```python
from build123d import *

# Parameters (mm, degrees)
F1_DEPTH = 13
F2_R     = 3


with BuildPart() as f1:
    # F0 (on Top) → F1 (new body)
    with BuildSketch(Plane.XY):
        with BuildLine():
            ThreePointArc((11.590273, 26.810686), (0, 6.40625), (-11.590273, 26.810686))
            Line((-11.590273, 26.810686), (-13.308113, 27.834907))
            ThreePointArc((-13.308113, 27.834907), (-14.957469, 15.858164), (-7.5, 6.342445))
            ThreePointArc((-7.5, 6.342445), (0, 4.40625), (7.5, 6.342445))
            ThreePointArc((7.5, 6.342445), (14.957469, 15.858164), (13.308113, 27.834907))
            Line((13.308113, 27.834907), (11.590273, 26.810686))
        make_face()
        with BuildLine():
            ThreePointArc((7.5, 6.342445), (0, 4.40625), (-7.5, 6.342445))
            Line((-7.5, 6.342445), (-7.5, -3.390785))
            ThreePointArc((-7.5, -3.390785), (-0.005535, -0.365641), (7.5, -3.363212))
            Line((7.5, -3.363212), (7.5, 6.342445))
        make_face()
        with BuildLine():
            ThreePointArc((7.5, -3.363212), (-0.005535, -0.365641), (-7.5, -3.390785))
            ThreePointArc((-7.5, -3.390785), (-10.644414, -9.208204), (-9.826055, -15.770215))
            Line((-9.826055, -15.770215), (-8.374253, -15.097704))
            ThreePointArc((-8.374253, -15.097704), (0.0144, -1.965623), (8.403054, -15.097704))
            Line((8.403054, -15.097704), (9.854855, -15.770215))
            ThreePointArc((9.854855, -15.770215), (10.669515, -9.188614), (7.5, -3.363212))
        make_face()
    extrude(amount=F1_DEPTH)

    # F2
    f2_edges = [f1.edges().sort_by_distance(p)[0] for p in [
        (7.5, 1.489616, 13),
        (-7.5, 1.47583, 13),
        (7.5, 1.489616, 0),
        (-7.5, 1.47583, 0),
    ]]
    fillet(f2_edges, radius=F2_R)


solid = f1.part
```
For this review, take the finished solid that the model builds, in its own axes (mm). A direction names the side the tool comes from. Coordinates: 2 decimals unless noted, no trailing zeros. Order: outer loops, then holes, each group sorted by start corner. A loop starts at its lowest first (then second) coordinate and runs counter-clockwise, first axis right, second up. Notation, with made-up numbers: (-4, 67.5) - (48, 67.5) arc R18 ccw to (48, 71.5) - close; hole circle Ø11 at (4, 44.5). An arc over 180 degrees is marked (long way). Answer as a JSON object with one key per item and string values. Group by question number.
1. We need section D-D on x = 5.5. State the section outline as (y, z) points.
2. We need section B-B on z = 8. State the section outline as (x, y) points, then the cut area to 3 significant figures.
3. We need section C-C on y = 2. State the section outline as (x, z) points.
4. For faces 1 (the cylindrical face through (-6.64, 1.41, 0.9)), 2 (the flat face through (7.5, 1, 6)), 3 (the cylindrical face through (6.64, 1.56, 12.1)), 4 (the flat face through (12.46, 27.33, 6.41)), 5 (the cylindrical face through (6.64, 1.56, 0.9)), list the 3-axis set-ups (+Z, -Z, +X, -X, +Y, -Y) from which the entire face can be reached by the end or side of a thin tool; tool diameter is ignored.
5. We need section A-A on y = -6.5. State the section outline as (x, z) points, then the cut area to 3 significant figures.
6. The part is to be moulded in two halves that separate along X. For faces 6 (the flat face through (-7.5, 2, 6)), 7 (the flat face through (9.12, -15.43, 6.41)), 8 (the cylindrical face through (15.243, 17.12, 6.409)), 9 (the flat face through (0, 6, 13)), say which applies: pulls with the +X half, pulls with the -X half, needs draft (parallel to the pull), parting line crosses it, or undercut.
7. For probe 1 along Y at (x, z) = (-8.5, 2.75); probe 2 along X at (y, z) = (20, 12); probe 3 along X at (y, z) = (-11.5, 1.25), list the stretches that pass through material, from the lowest coordinate up.
8. Clearance check with flat-ended pins moving along their axes: P1, Ø5, axis at y = -6.5, z = 2.5, coming from the +X side; P2, Ø7.5, axis at y = 1.5, z = 6, coming from the +X side; P3, Ø2, axis at y = 11, z = 8, coming from the +X side. State where each tip first meets the part, or that it passes through.
Final values:
{
 "1": {"outline": "(-3.77, 0) - (-1.86, 0) - (-1.86, 0.17) - (5.42, 0.17) - (5.42, 0) - (7.58, 0) - (7.58, 13) - (5.42, 13) - (5.42, 12.83) - (-1.86, 12.83) - (-1.86, 13) - (-3.77, 13) - close"},
 "2": {"outline": "(-13.31, 27.83) arc R15.49 ccw to (-7.5, 6.34) - (-7.5, -3.39) arc R10.85 ccw to (-9.83, -15.77) - (-8.37, -15.1) arc R9.25 cw (long way) to (8.4, -15.1) - (9.85, -15.77) arc R10.85 ccw to (7.5, -3.36) - (7.5, 6.34) arc R15.49 ccw to (13.31, 27.83) - (11.59, 26.81) arc R13.49 cw (long way) to (-11.59, 26.81) - close", "area": "282 mm²"},
 "3": {"outline": "(-7.5, 3) arc R3 ccw to (-4.5, 0) - (4.5, 0) arc R3 ccw to (7.5, 3) - (7.5, 10) arc R3 ccw to (4.5, 13) - (-4.5, 13) arc R3 ccw to (-7.5, 10) - close"},
 "4": {"face 1": "-Z, -X", "face 2": "+Z, -Z, +X", "face 3": "+Z, +X", "face 4": "+Z, -Z, +Y", "face 5": "-Z, +X"},
 "5": {"outline": "(-9.75, 0) - (-7.94, 0) - (-7.94, 13) - (-9.75, 13) - close; (7.97, 0) - (9.78, 0) - (9.78, 13) - (7.97, 13) - close", "area": "47.2 mm²"},
 "6": {"face 6": "pulls with the -X half", "face 7": "undercut", "face 8": "pulls with the +X half", "face 9": "needs draft"},
 "7": {"probe 1": "-15.16 to -14.81, -7.61 to -4.49, 6.95 to 9.42", "probe 2": "-15.49 to -13.49, 13.49 to 15.49", "probe 3": "-10.83 to -9.23, 9.26 to 10.86"},
 "8": {"P1": "x = 10.63", "P2": "x = 7.5", "P3": "x = 13.33"}
}
